from build123d import *

# Parameters (mm, degrees)
F0_W        = 80
F0_H        = 40
F0_R        = 3
F0_W_2      = 50
F0_H_2      = 30
F1_DEPTH    = 5
F2_SIZE     = 2
F6_DEPTH    = 40
F7_T1_DEPTH = 40
F7_T3_DEPTH = 64.9354908843
F7_T5_DEPTH = 47.905041839


# Not quite as in the source:
# - a fillet or chamfer that OpenCascade refuses, or shapes differently, is made with other operations: its cross-section is extruded or revolved along the edge and cut away or added


with BuildPart() as f1:
    # F0 (on Top) → F1 (new body)
    with BuildSketch(Plane.XY):
        with Locations((40, -20)):
            Rectangle(F0_W, F0_H)
        with Locations((7.5, -20)):
            Circle(F0_R, mode=Mode.SUBTRACT)
        with Locations((40, -20)):
            Rectangle(F0_W_2, F0_H_2, mode=Mode.SUBTRACT)
        with Locations((72.5, -20)):
            Circle(F0_R, mode=Mode.SUBTRACT)
        with Locations((40, -20)):
            Rectangle(F0_W_2, F0_H_2)
    extrude(amount=F1_DEPTH)

    # F2
    f2_edges = [f1.edges().sort_by_distance(p)[0] for p in [
        (4.5, -20, 5),
        (69.5, -20, 5),
    ]]
    chamfer(f2_edges, length=F2_SIZE)

    # F5 (on plane+point) → F6 (join)
    with BuildSketch(Plane(origin=(0, 0, 0), x_dir=(-1, 0, 0), z_dir=(0, 1, 0))):
        with BuildLine():
            ThreePointArc((-30.954095751, 30.0433963806), (-37.954095751, 5), (-44.954095751, 30.0433963806))
            Line((-44.954095751, 30.0433963806), (-44.954095751, 39.8834047803))
            ThreePointArc((-44.954095751, 39.8834047803), (-58.6775836128, 27.2628220822), (-58.1714250849, 8.625305341))
            Line((-58.1714250849, 8.625305341), (-58.1714250849, 0))
            Line((-58.1714250849, 0), (-17.7367664172, 0))
            Line((-17.7367664172, 0), (-17.7367664172, 8.625305341))
            ThreePointArc((-17.7367664172, 8.625305341), (-17.2306078893, 27.2628220822), (-30.954095751, 39.8834047803))
            Line((-30.954095751, 39.8834047803), (-30.954095751, 30.0433963806))
        make_face()
    extrude(amount=-F6_DEPTH)

    # F7: fillet of radius 3 on 8 edges, made by hand

    # F7_s2 → F7_t1 (join)
    with BuildSketch(Plane.XZ):
        with BuildLine():
            ThreePointArc((58.1714250849, 7.9545925349), (58.2393309928, 8.5892768936), (58.439974575, 9.1952287073))
            ThreePointArc((58.439974575, 9.1952287073), (58.3076947386, 8.9093270176), (58.1714250849, 8.625305341))
            Line((58.1714250849, 8.625305341), (58.1714250849, 7.9545925349))
        make_face()
        with BuildLine():
            ThreePointArc((61.1714250849, 5), (59.0501047413, 5.8786796564), (58.1714250849, 8))
            Line((58.1714250849, 8), (58.1714250849, 5))
            Line((58.1714250849, 5), (61.1714250849, 5))
        make_face()
        with BuildLine():
            ThreePointArc((17.4682169271, 9.1952287073), (17.6688605093, 8.5892768936), (17.7367664172, 7.9545925349))
            Line((17.7367664172, 7.9545925349), (17.7367664172, 8.625305341))
            ThreePointArc((17.7367664172, 8.625305341), (17.6004967635, 8.9093270176), (17.4682169271, 9.1952287073))
        make_face()
        with BuildLine():
            ThreePointArc((17.7367664172, 8), (16.8580867608, 5.8786796564), (14.7367664172, 5))
            Line((14.7367664172, 5), (17.7367664172, 5))
            Line((17.7367664172, 5), (17.7367664172, 8))
        make_face()
    extrude(amount=F7_T1_DEPTH)

    # F7_s4 → F7_t3 (cut)
    with BuildSketch(Plane.XZ.offset(-12.4677454421)):
        with BuildLine():
            ThreePointArc((44.954095751, 35.2406690428), (46.4734514007, 37.8498245207), (49.4925572895, 37.8161565878))
            ThreePointArc((49.4925572895, 37.8161565878), (47.2807788606, 38.9759122428), (44.954095751, 39.8834047803))
            Line((44.954095751, 39.8834047803), (44.954095751, 35.2406690428))
        make_face()
        with BuildLine():
            ThreePointArc((26.4156342126, 37.8161565878), (29.4347401014, 37.8498245207), (30.954095751, 35.2406690428))
            Line((30.954095751, 35.2406690428), (30.954095751, 39.8834047803))
            ThreePointArc((30.954095751, 39.8834047803), (28.6274126415, 38.9759122428), (26.4156342126, 37.8161565878))
        make_face()
    extrude(amount=F7_T3_DEPTH, mode=Mode.SUBTRACT)

    # F7_s6 → F7_t5 (cut)
    with BuildSketch(Plane.XZ.offset(-3.9525209195)):
        with BuildLine():
            ThreePointArc((46.1359139329, 29.2381493396), (45.2657370088, 30.2929667015), (44.954095751, 31.6244047484))
            Line((44.954095751, 31.6244047484), (44.954095751, 30.0433963806))
            ThreePointArc((44.954095751, 30.0433963806), (45.5556749637, 29.6564328293), (46.1359139329, 29.2381493396))
        make_face()
        with BuildLine():
            ThreePointArc((30.954095751, 31.6244047484), (30.6424544933, 30.2929667015), (29.7722775692, 29.2381493396))
            ThreePointArc((29.7722775692, 29.2381493396), (30.3525165384, 29.6564328293), (30.954095751, 30.0433963806))
            Line((30.954095751, 30.0433963806), (30.954095751, 31.6244047484))
        make_face()
    extrude(amount=F7_T5_DEPTH, mode=Mode.SUBTRACT)


solid = f1.part
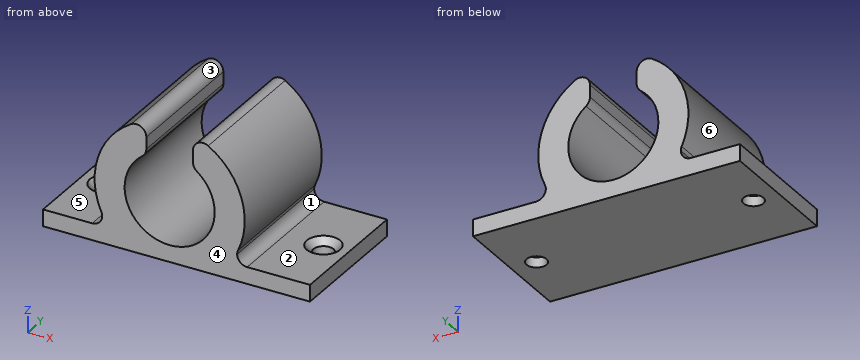
For this review, take the finished solid that the model builds, in its own axes (mm). Face numbers are marked on the shaded views. A direction names the side the tool comes from. Round coordinates to 2 decimals unless told otherwise and drop trailing zeros. Write each loop counter-clockwise with the first axis right and the second up, starting at its lowest first coordinate (ties: lowest second). Pieces come first, ordered by that corner, then holes. Notation, with made-up numbers: M 0,21.5 L 52,21.5 A19 cw 52,55.5 Z; hole C 12,24 d6. An arc over 180 degrees is marked long. Write item = value, one per line. Start each with the question number.
(1) For the marked faces 1, 2 and 3, list the 3-axis set-ups (+Z, -Z, +X, -X, +Y, -Y) from which the entire face can be reached by the end or side of a thin tool; tool diameter is ignored.
(2) For line 1 along Y through (x, z) = (72.5, 1.7); line 2 along Z through (x, y) = (72.5, -2.5); line 3 along Z through (x, y) = (58.5, -9), list the stretches that pass through material, from the lowest coordinate up.
(3) We need section D-D (y = -35). Give the boundary of the cut face in (x, z).
(4) We need section C-C (z = 15.5). Give the boundary of the cut face in (x, y) (3 decimals), then the cut area to 3 significant figures.
(5) We need section A-A (y = -20). Give the number of separate pieces and of enclosed holes in the cut face, then the cut area to 3 significant figures.
(6) The part is to be moulded in two halves that separate along Z. For the marked faces 4, 5 and 6, say which applies: +Z half, -Z half, draft (parallel to the pull), parting line (faces both ways), or undercut.
(7) We need section B-B (x = 7.5). Give the boundary of the cut face in (y, z), then the cut area to 3 significant figures.
(8) Clearance check with flat-ended pins moving along their axes: pin 1 Ø12 at (y, z) = (-5, 21.5) entering from +X; pin 2 Ø2 at (y, z) = (-34, 28.5) entering from +X; pin 3 Ø1 at (x, y) = (23.5, -35) entering from -Z; pin 4 Ø3 at (x, y) = (69.5, -29) entering from +Z. State where each tip first meets the part, or that it passes through.
Results found:
q1.face_1 = +X, +Y, -Y
q1.face_2 = +Z, +X, +Y, -Y
q1.face_3 = +Z, +Y, -Y
q2.line_1 = -40 to -23, -17 to 0
q2.line_2 = 0 to 5
q2.line_3 = 0 to 6.63, 9.33 to 27.67
q3.outline = M 0,0 L 80,0 L 80,5 L 61.17,5 A3 cw 58.17,7.98 A3 cw 58.44,9.2 A22.5 ccw 49.49,37.82 A3 ccw 44.95,35.24 L 44.95,31.62 A3 ccw 46.14,29.24 A13.5 cw long 29.77,29.24 A3 ccw 30.95,31.62 L 30.95,35.24 A3 ccw 26.42,37.82 A22.5 ccw 17.47,9.2 A3 cw 17.74,7.98 A3 cw 14.74,5 L 0,5 Z
q4.outline = M 15.655,-40 L 24.792,-40 L 24.792,0 L 15.655,0 Z; M 51.117,-40 L 60.253,-40 L 60.253,0 L 51.117,0 Z
q4.area = 731 mm²
q5.separate_pieces = 3
q5.enclosed_holes = 0
q5.area = 994 mm²
q6.face_4 = draft
q6.face_5 = +Z half
q6.face_6 = undercut
q7.outline = M -40,0 L -23,0 L -23,3 L -25,5 L -40,5 Z; M -17,0 L 0,0 L 0,5 L -15,5 L -17,3 Z
q7.area = 166 mm²
q8.pin_1 = 60.45
q8.pin_2 = 58.58
q8.pin_3 = 0
q8.pin_4 = 5
